Part model, mm, in its own coordinate system. A direction names the side the tool comes from. Round coordinates to 2 decimals unless told otherwise and drop trailing zeros. Write each loop counter-clockwise with the first axis right and the second up, starting at its lowest first coordinate (ties: lowest second). Pieces come first, ordered by that corner, then holes. Notation, with made-up numbers: (-10.5, 43.5) -> (46.5, 43.5) arc R24 cw to (46.5, 72.5) -> close; hole circle Ø3 at (-18.5, 19.5). An arc over 180 degrees is marked (long way). Return JSON: item names as keys, results as strings. Group by question number.
(1) Drop flat-ended pins along their axis: pin 1 Ø8 at (x, y) = (26, 13.5) entering from -Z; pin 2 Ø2 at (x, y) = (-20, 37.5) entering from -Z; pin 3 Ø2 at (x, y) = (-24, -38) entering from +Z; pin 4 Ø0.7 at (y, z) = (36, 3) entering from +X. Give the stop position or say it passes through.
(2) Saw through at A-A (y = -34.5). List the corners of the cut face in (x, z), plus the area to 3 significant figures.
(3) Mould opens along Z. For faces 5 (the flat face through (23, -38, 13.5)), 6 (the flat face through (-38, -3, 17)), 7 (the flat face through (32, 34, 11)) say: +Z half, -Z half, draft (parallel to the pull), parting line (faces both ways), or undercut.
(4) Saw through at D-D (y = -10.2). List the corners of the cut face in (x, z), plus the area to 3 significant figures.
(5) Tool access for faces 1 (the flat face through (32, -35, 11)), 2 (the cylindrical face through (-38.014, 2.662, 15.553)), 3 (the flat face through (23, 38, 10.5)), 4 (the flat face through (0, 37.5, 6)): list every direction of +Z, -Z, +X, -X, +Y, -Y with a clear straight run to the whole face (end or side of a thin tool).
(6) Drill centre lines: L1, parallel to X at y = 34.5, z = 10.75; L2, parallel to Y at x = -2, z = 15.5. Where is each one in solid material? Low to high. Write a range as from..to.
(7) Saw through at C-C (z = 2). List the corners of the cut face in (x, y), plus the area to 3 significant figures.
(8) Saw through at B-B (x = 20). State how many separate pieces and enclosed holes the cut face has, plus the area to 4 significant figures.
from build123d import *

# Parameters (mm, degrees)
SKETCH_1_W           = 78
SKETCH_1_H           = 78
EXTRUDE_1_DEPTH      = 6
SKETCH_2_W           = 78
SKETCH_2_H           = 78
SKETCH_2_W_2         = 74
SKETCH_2_H_2         = 74
SKETCH_2_W_3         = 5
SKETCH_2_H_3         = 5
EXTRUDE_2_DEPTH      = 11
FILLET_1_R           = 1.5
FILLET_2_R           = 3.5
CUT_EXTRUDE_1_DEPTH  = 1
CUT_EXTRUDE_2_DEPTH  = 3
SKETCH_5_R           = 1.15
CUT_EXTRUDE_3_DEPTH  = 58.428216061
SKETCH_6_W           = 55
SKETCH_6_H           = 2
SKETCH_6_W_2         = 54
SKETCH_6_H_2         = 58
SKETCH_6_W_3         = 12.5
SKETCH_6_H_3         = 42
CUT_EXTRUDE_4_DEPTH  = 57.665686266
EXTRUDE_3_DEPTH      = 1
EXTRUDE_3_DEPTH_BACK = 2
SKETCH_7_W           = 10
SKETCH_7_H           = 1.5
SKETCH_7_W_2         = 28
SKETCH_8_R           = 4.25
SKETCH_8_R_2         = 2.247220505
CUT_EXTRUDE_5_DEPTH  = 10
CUT_EXTRUDE_6_DEPTH  = 90.044932478
SKETCH_10_W          = 1.3
SKETCH_10_H          = 2.3
CUT_EXTRUDE_7_DEPTH  = 3


with BuildPart() as part:
    # 草图1 → 凸台-拉伸1 (new body)
    with BuildSketch(Plane.XY):
        Rectangle(SKETCH_1_W, SKETCH_1_H)
    extrude(amount=EXTRUDE_1_DEPTH)

    # 草图2 → 凸台-拉伸2 (add)
    # profile 1 of 5: a face of its own
    with BuildSketch(Plane.XY.offset(6)):
        Rectangle(SKETCH_2_W, SKETCH_2_H)
        Rectangle(SKETCH_2_W_2, SKETCH_2_H_2, mode=Mode.SUBTRACT)
    # profile 2 of 5: a face of its own
    with BuildSketch(Plane.XY.offset(6)):
        with Locations((-34.5, 34.5)):
            Rectangle(SKETCH_2_W_3, SKETCH_2_H_3)
    # profile 3 of 5: a face of its own
    with BuildSketch(Plane.XY.offset(6)):
        with Locations((34.5, 34.5)):
            Rectangle(SKETCH_2_W_3, SKETCH_2_H_3)
    # profile 4 of 5: a face of its own
    with BuildSketch(Plane.XY.offset(6)):
        with Locations((34.5, -34.5)):
            Rectangle(SKETCH_2_W_3, SKETCH_2_H_3)
    # profile 5 of 5: a face of its own
    with BuildSketch(Plane.XY.offset(6)):
        with Locations((-34.5, -34.5)):
            Rectangle(SKETCH_2_W_3, SKETCH_2_H_3)
    extrude(amount=EXTRUDE_2_DEPTH)

    # 圆角1
    fillet_1_edges = [part.edges().sort_by_distance(p)[0] for p in [
        (-37, -32, 11.5),
        (-37, 32, 11.5),
        (-32, 32, 11.5),
        (-32, 37, 11.5),
        (32, 37, 11.5),
        (32, 32, 11.5),
        (37, 32, 11.5),
        (37, -32, 11.5),
        (32, -32, 11.5),
        (32, -37, 11.5),
        (-32, -37, 11.5),
        (-32, -32, 11.5),
    ]]
    fillet(fillet_1_edges, radius=FILLET_1_R)

    # 圆角2
    fillet_2_edges = [part.edges().sort_by_distance(p)[0] for p in [
        (39, -39, 8.5),
        (-39, -39, 8.5),
        (-39, 39, 8.5),
        (39, 39, 8.5),
    ]]
    fillet(fillet_2_edges, radius=FILLET_2_R)

    # 草图3 → 切除-拉伸1 (cut)
    with BuildSketch(Plane(origin=(0, 0, 0), x_dir=(-1, 0, 0), z_dir=(0, 0, -1))):
        with BuildLine():
            Line((37.5, -35.5), (37.5, 35.5))
            ThreePointArc((37.5, 35.5), (36.914213562, 36.914213562), (35.5, 37.5))
            Line((35.5, 37.5), (-35.5, 37.5))
            ThreePointArc((-35.5, 37.5), (-36.914213562, 36.914213562), (-37.5, 35.5))
            Line((-37.5, 35.5), (-37.5, -35.5))
            ThreePointArc((-37.5, -35.5), (-36.914213562, -36.914213562), (-35.5, -37.5))
            Line((-35.5, -37.5), (35.5, -37.5))
            ThreePointArc((35.5, -37.5), (36.914213562, -36.914213562), (37.5, -35.5))
        make_face()
    extrude(amount=-CUT_EXTRUDE_1_DEPTH, mode=Mode.SUBTRACT)

    # 草图4 → 切除-拉伸2 (cut)
    with BuildSketch(Plane(origin=(0, 0, 1), x_dir=(-1, 0, 0), z_dir=(0, 0, -1))):
        Polygon((27.5, 37.5), (-27.5, 37.5), (-27.5, 37.1), (-33.2, 37.1), (-33.2, -33.5), (33.2, -33.5), (33.2, 37.1), (27.5, 37.1), align=None)
    extrude(amount=-CUT_EXTRUDE_2_DEPTH, mode=Mode.SUBTRACT)

    # 草图5 → 切除-拉伸3 (cut, through all)
    with BuildSketch(Plane(origin=(0, 0, 1), x_dir=(-1, 0, 0), z_dir=(0, 0, -1))):
        with Locations((-34.5, 34.5)):
            Circle(SKETCH_5_R)
        with Locations((34.5, 34.5)):
            Circle(SKETCH_5_R)
        with Locations((34.5, -34.5)):
            Circle(SKETCH_5_R)
        with Locations((-34.5, -34.5)):
            Circle(SKETCH_5_R)
    extrude(amount=-CUT_EXTRUDE_3_DEPTH, mode=Mode.SUBTRACT)

    # 草图6 → 切除-拉伸4 (cut, through all)
    with BuildSketch(Plane(origin=(0, 0, 4), x_dir=(-1, 0, 0), z_dir=(0, 0, -1))):
        with Locations((0, 36.5)):
            Rectangle(SKETCH_6_W, SKETCH_6_H)
        with Locations((9, 1)):
            Rectangle(SKETCH_6_W_2, SKETCH_6_H_2)
        with Locations((-28.75, -5)):
            Rectangle(SKETCH_6_W_3, SKETCH_6_H_3)
    extrude(amount=-CUT_EXTRUDE_4_DEPTH, mode=Mode.SUBTRACT)

    # 草图7 → 凸台-拉伸3 (add, two sides: drawn at the far end of the back side and taken through both)
    with BuildSketch(Plane.XY.offset(17).offset(-EXTRUDE_3_DEPTH_BACK)):
        with Locations((9, -36.75)):
            Rectangle(SKETCH_7_W, SKETCH_7_H)
        with Locations((-9, -36.75)):
            Rectangle(SKETCH_7_W, SKETCH_7_H)
        with Locations((0, 36.75)):
            Rectangle(SKETCH_7_W_2, SKETCH_7_H)
    extrude(amount=EXTRUDE_3_DEPTH + EXTRUDE_3_DEPTH_BACK)

    # 草图8 → 切除-拉伸5 (cut)
    with BuildSketch(Plane(origin=(-39, 0, 0), x_dir=(0, 0, -1), z_dir=(1, 0, 0))):
        with Locations((-16.5, -10.2)):
            Circle(SKETCH_8_R)
        with Locations((-17.8, 2.7)):
            Circle(SKETCH_8_R_2)
    extrude(amount=CUT_EXTRUDE_5_DEPTH, mode=Mode.SUBTRACT)

    # 草图9 → 切除-拉伸6 (cut, through all)
    with BuildSketch(Plane.XZ.offset(39)):
        with BuildLine():
            Line((-29, 15.5), (-17, 15.5))
            ThreePointArc((-17, 15.5), (-16, 14.5), (-17, 13.5))
            Line((-17, 13.5), (-29, 13.5))
            ThreePointArc((-29, 13.5), (-30, 14.5), (-29, 15.5))
        make_face()
        with BuildLine():
            Line((-29, 10.5), (-17, 10.5))
            ThreePointArc((-17, 10.5), (-16, 9.5), (-17, 8.5))
            Line((-17, 8.5), (-29, 8.5))
            ThreePointArc((-29, 8.5), (-30, 9.5), (-29, 10.5))
        make_face()
        with BuildLine():
            Line((29, 10.5), (17, 10.5))
            ThreePointArc((17, 10.5), (16, 9.5), (17, 8.5))
            Line((17, 8.5), (29, 8.5))
            ThreePointArc((29, 8.5), (30, 9.5), (29, 10.5))
        make_face()
        with BuildLine():
            Line((29, 15.5), (17, 15.5))
            ThreePointArc((17, 15.5), (16, 14.5), (17, 13.5))
            Line((17, 13.5), (29, 13.5))
            ThreePointArc((29, 13.5), (30, 14.5), (29, 15.5))
        make_face()
    extrude(amount=-CUT_EXTRUDE_6_DEPTH, mode=Mode.SUBTRACT)

    # 草图10 → 切除-拉伸7 (cut)
    with BuildSketch(Plane(origin=(0, 0, 1), x_dir=(-1, 0, 0), z_dir=(0, 0, -1))):
        with Locations((-33.85, 34.5)):
            Rectangle(SKETCH_10_W, SKETCH_10_H)
        with Locations((33.85, 34.5)):
            Rectangle(SKETCH_10_W, SKETCH_10_H)
    extrude(amount=-CUT_EXTRUDE_7_DEPTH, mode=Mode.SUBTRACT)


solid = part.part
Computed values:
{
 "1": {"pin 1": "z = 4", "pin 2": "z = 0", "pin 3": "z = 17", "pin 4": "x = 39"},
 "2": {"outline": "(-39, 0) -> (-37.5, 0) -> (-37.5, 1) -> (-35.65, 1) -> (-35.65, 17) -> (-39, 17) -> close; (-33.35, 1) -> (33.35, 1) -> (33.35, 17) -> (32, 17) -> (32, 6) -> (-32, 6) -> (-32, 17) -> (-33.35, 17) -> close; (35.65, 1) -> (37.5, 1) -> (37.5, 0) -> (39, 0) -> (39, 17) -> (35.65, 17) -> close", "area": "473 mm2"},
 "3": {"face 5": "undercut", "face 6": "+Z half", "face 7": "draft"},
 "4": {"outline": "(-39, 0) -> (-37.5, 0) -> (-37.5, 1) -> (-33.2, 1) -> (-33.2, 4) -> (-36, 4) -> (-36, 6) -> (-37, 6) -> (-37, 12.25) -> (-39, 12.25) -> close; (18, 4) -> (22.5, 4) -> (22.5, 6) -> (18, 6) -> close; (33.2, 1) -> (37.5, 1) -> (37.5, 0) -> (39, 0) -> (39, 17) -> (37, 17) -> (37, 6) -> (35, 6) -> (35, 4) -> (33.2, 4) -> close", "area": "95.3 mm2"},
 "5": {"face 1": "+Z", "face 2": "+Z, -X", "face 3": "+Y, -Y", "face 4": "-Z"},
 "6": {"L1": "-39..-35.65, -33.35..-32, 32..33.35, 35.65..39", "L2": "-39..-37, 36..39"},
 "7": {"outline": "(-39, -35.5) arc R3.5 ccw to (-35.5, -39) -> (35.5, -39) arc R3.5 ccw to (39, -35.5) -> (39, 35.5) arc R3.5 ccw to (35.5, 39) -> (-35.5, 39) arc R3.5 ccw to (-39, 35.5) -> close; hole circle Ø2.3 at (-34.5, -34.5); hole (-34.5, 33.35) -> (-33.2, 33.35) -> (-33.2, -33.5) -> (33.2, -33.5) -> (33.2, 33.35) -> (34.5, 33.35) arc R1.15 ccw to (34.5, 35.65) -> (33.2, 35.65) -> (33.2, 37.1) -> (27.5, 37.1) -> (27.5, 37.5) -> (-27.5, 37.5) -> (-27.5, 37.1) -> (-33.2, 37.1) -> (-33.2, 35.65) -> (-34.5, 35.65) arc R1.15 ccw to start; hole circle Ø2.3 at (34.5, -34.5)", "area": "1,350 mm2"},
 "8": {"separate pieces": "6", "enclosed holes": "0", "area": "200.5 mm2"}
}
